Input: dimensioned drawing with shaded views. Units: mm. Origin: part minimum x, y, z. A direction names the side the tool comes from. Give positions to 0.01 mm unless a question says otherwise; leave off trailing zeros. Write each loop counter-clockwise with the first axis right and the second up, starting at its lowest first coordinate (ties: lowest second). Pieces come first, ordered by that corner, then holes.
Q1. Section A-A (x = 33.5). Return the cut outline in (y, z) (1 decimal), plus the area to 3 significant figures.
Q2. Mould query, pull axis X, two halves, no side actions, for the marked faces 6, 7 and 8. Classes: +X half, -X half, draft (parallel to the pull), parting line (faces both ways), or undercut.
Q3. Reachability of the marked faces 1, 2, 3, 4 and 5 from +Z, -Z, +X, -X, +Y, -Y: full face, straight path, thin tool, end or side. Return the list, or none.
Q4. Section D-D (x = 47.5). Return the cut outline in (y, z), plus the area to 3 significant figures.
Q5. Line query: line 1 (Z direction, x = 54, y = 40); line 2 (X direction, y = 12, z = 10). Output: solid intervals per line, ascending.
Q6. Pin query (flat end, axial travel): pin 1 Ø20.5 at (x, z) = (60, 31.5) entering from -Y; pin 2 Ø5 at (x, y) = (42, 11.5) entering from +Z; pin 3 Ø1.5 at (y, z) = (38.5, 52.5) entering from +X; pin 4 Ø1.5 at (y, z) = (11, 8.5) entering from +X. Return the tip coordinate at first contact, or that it passes through.
Q7. Section B-B (z = 20.5). Return the cut outline in (x, y) (1 decimal), plus the area to 3 significant figures.
Q8. Section C-C (y = 23). Return the cut outline in (x, z).
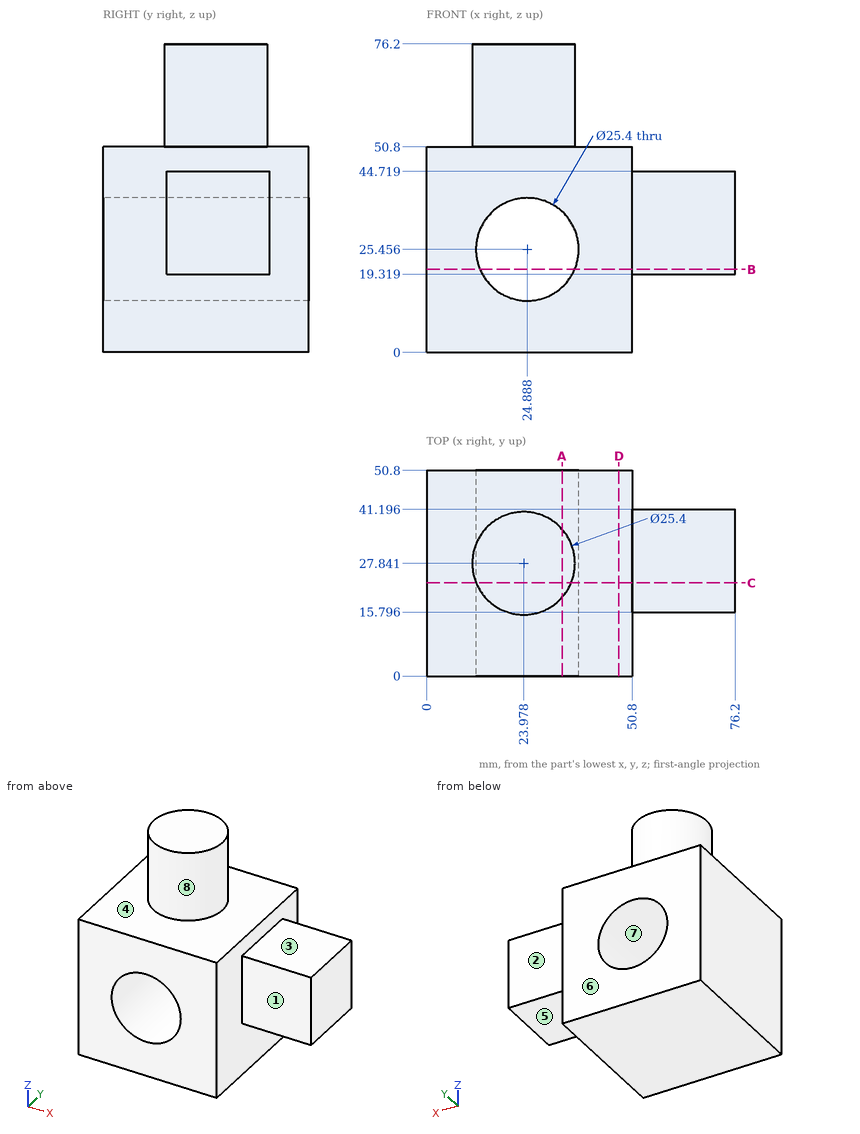
Computed:
1. outline: (0, 0) - (50.8, 0) - (50.8, 16.1) - (0, 16.1) - close; (0, 34.8) - (50.8, 34.8) - (50.8, 50.8) - (36.2, 50.8) - (36.2, 76.2) - (19.4, 76.2) - (19.4, 50.8) - (0, 50.8) - close
1. area: 2,060 mm2
2. face 6: draft
2. face 7: undercut
2. face 8: parting line
3. face 1: +Z, -Z, +X, -Y
3. face 2: +Z, -Z, +X, +Y
3. face 3: +Z, +X, +Y, -Y
3. face 4: +Z
3. face 5: -Z, +X, +Y, -Y
4. outline: (0, 0) - (50.8, 0) - (50.8, 50.8) - (0, 50.8) - close
4. area: 2,580 mm2
5. line 1: z = 19.32 to 44.72
5. line 2: x = 0 to 50.8
6. pin 1: stops at y = 0
6. pin 2: stops at z = 50.8
6. pin 3: stops at x = 31.92
6. pin 4: stops at x = 50.8
7. outline: (0, 0) - (13.2, 0) - (13.2, 50.8) - (0, 50.8) - close; (36.6, 0) - (50.8, 0) - (50.8, 15.8) - (76.2, 15.8) - (76.2, 41.2) - (50.8, 41.2) - (50.8, 50.8) - (36.6, 50.8) - close
7. area: 2,040 mm2
8. outline: (0, 0) - (50.8, 0) - (50.8, 19.32) - (76.2, 19.32) - (76.2, 44.72) - (50.8, 44.72) - (50.8, 50.8) - (35.72, 50.8) - (35.72, 76.2) - (12.24, 76.2) - (12.24, 50.8) - (0, 50.8) - close; hole circle Ø25.4 at (24.89, 25.46)
